Input: dimensioned drawing with shaded views. Units: mm. Origin: part minimum x, y, z. A direction names the side the tool comes from. Give positions to 0.01 mm unless a question says otherwise; leave off trailing zeros. Loops run counter-clockwise (first coordinate to the right, second up) from the corner with the lowest first, then second, coordinate; pieces in that order, holes last. Notation, with made-up numbers: (0.5, -27.5) -> (28.5, -27.5) arc R14 cw to (28.5, -8.5) -> close; hole circle Ø5 at (76.25, 4). An arc over 180 degrees is marked (long way). Answer as a JSON object with one key per item and string values.
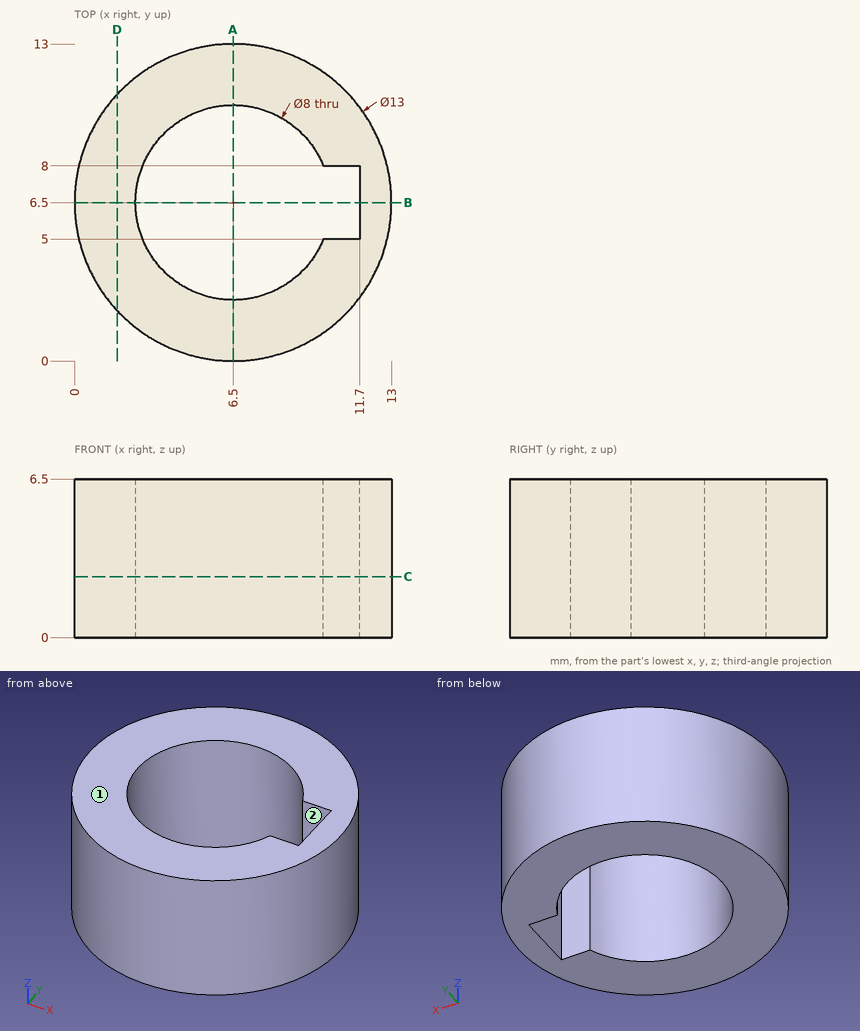
Q1. Ray query, line 1 along Y through (x, z) = (6.5, 3.25); line 2 along X through (y, z) = (5.75, 4.75); line 3 along Y through (x, z) = (8.25, 2.25). Return the intervals inside material, ascending.
Evaluation:
{"line 1": "y = 0 to 2.5, 10.5 to 13", "line 2": "x = 0.04 to 2.57, 11.7 to 12.96", "line 3": "y = 0.24 to 2.9, 10.1 to 12.76"}
Q2. Access query for the marked faces 1 and 2. Directions: +Z, -Z, +X, -X, +Y, -Y. A direction counts if a zero-diameter tool reaches every point of the face in a straight line with its end or side. Return the directions, or none.
Evaluation:
{"face 1": "+Z, +X, -X, +Y, -Y", "face 2": "+Z, -Z"}
Q3. Pin query (flat end, axial travel): pin 1 (2 mm diameter, centred on x = 8, z = 5.5, fed in from -Y); pin 2 (1.5 mm diameter, centred on y = 7.5, z = 0.5, fed in from -X); pin 3 (1 mm diameter, centred on x = 3, z = 1.5, fed in from +Y); pin 4 (7 mm diameter, centred on x = 6.5, y = 6.5, fed in from -Z). Return the tip coordinate at first contact, or that it passes through.
Evaluation:
{"pin 1": "stops at y = 0.02", "pin 2": "stops at x = 0", "pin 3": "stops at y = 12.27", "pin 4": "passes through"}
Q4. Section A-A, the plane x = 6.5. Return the cut outline in (y, z), then the cut area to 3 significant figures.
Evaluation:
{"outline": "(0, 0) -> (2.5, 0) -> (2.5, 6.5) -> (0, 6.5) -> close; (10.5, 0) -> (13, 0) -> (13, 6.5) -> (10.5, 6.5) -> close", "area": "32.5 mm2"}
Q5. Section D-D, the plane x = 1.75. Return the cut outline in (y, z).
Evaluation:
{"outline": "(2.06, 0) -> (10.94, 0) -> (10.94, 6.5) -> (2.06, 6.5) -> close"}
Q6. Section C-C, the plane z = 2.5. Return the cut outline in (x, y).
Evaluation:
{"outline": "circle Ø13 at (6.5, 6.5); hole (10.21, 5) -> (11.7, 5) -> (11.7, 8) -> (10.21, 8) arc R4 ccw (long way) to start"}
Q7. Section B-B, the plane y = 6.5. Return the cut outline in (x, z), then the cut area to 3 significant figures.
Evaluation:
{"outline": "(0, 0) -> (2.5, 0) -> (2.5, 6.5) -> (0, 6.5) -> close; (11.7, 0) -> (13, 0) -> (13, 6.5) -> (11.7, 6.5) -> close", "area": "24.7 mm2"}
